The model under review builds one solid part; all positions refer to its coordinate system, in mm. Coordinates: 2 decimals unless noted, no trailing zeros. Loops run counter-clockwise (first coordinate to the right, second up) from the corner with the lowest first, then second, coordinate; pieces in that order, holes last. Notation, with made-up numbers: M 26.25,-21 L 64.25,-21 A20 ccw 64.25,-7 Z; hole C 27,-34 d5. An arc over 180 degrees is marked long. One line per item, written item: value.
```python
from build123d import *

# Parameters (mm, degrees)
SKETCH1_R           = 25
BOSS_EXTRUDE1_DEPTH = 1050
SKETCH2_W           = 20
SKETCH2_H           = 15
BOSS_EXTRUDE2_DEPTH = 200


with BuildPart() as part:
    # Sketch1 → Boss-Extrude1 (new body)
    with BuildSketch(Plane(origin=(0, 0, 0), x_dir=(0, 0, -1), z_dir=(1, 0, 0))):
        Circle(SKETCH1_R)
    extrude(amount=BOSS_EXTRUDE1_DEPTH)

    # Sketch2 → Boss-Extrude2 (add)
    with BuildSketch(Plane.ZY.offset(-325)):
        with Locations((0, 30.412878475)):
            Rectangle(SKETCH2_W, SKETCH2_H)
    extrude(amount=-BOSS_EXTRUDE2_DEPTH)


solid = part.part
```
(1) To check wall thickness, follow L1, parallel to Z at x = 770, y = 23; L2, parallel to Y at x = 53, z = 1; L3, parallel to Y at x = 967.5, z = 3. State the ranges of each line that lie inside material, in increasing order. Write a range as [from, to].
Checks:
L1: [-9.8, 9.8]
L2: [-24.98, 24.98]
L3: [-24.82, 24.82]
(2) Add section B-B on x = 972.5. State the section outline as (y, z) points.
Checks:
outline: C 0,0 d50
(3) Add section A-A on z = 0. State the section outline as (x, y) points.
Checks:
outline: M 0,-25 L 1050,-25 L 1050,25 L 525,25 L 525,37.91 L 325,37.91 L 325,25 L 0,25 Z
(4) Add section D-D on x = 396. State the section outline as (y, z) points, then the cut area to 3 significant figures.
Checks:
outline: M 22.91,-10 L 37.91,-10 L 37.91,10 L 22.91,10 A25 ccw long Z
area: 2,240 mm^2
(5) Add section C-C on y = -14. State the section outline as (x, z) points.
Checks:
outline: M 0,-20.71 L 1050,-20.71 L 1050,20.71 L 0,20.71 Z
(6) Insertion check: pin 1 Ø1.5 at (x, z) = (580, -9) entering from -Y; pin 2 Ø12 at (x, z) = (942, -8) entering from -Y; pin 3 Ø5 at (x, z) = (552, 1) entering from +Y. Each pin has a flat end and moves straight along its axis. Give the tip position at first contact, or say it passes through.
Checks:
pin 1: y = -23.6
pin 2: y = -24.92
pin 3: y = 25
